from build123d import *

# Parameters (mm, degrees)
F0_W     = 1044
F0_H     = 389
F1_DEPTH = 288
F2_R     = 100
F4_DEPTH = 389.001
F5_R     = 15
F6_DEPTH = 50


with BuildPart() as f1:
    # F0 (on Front) → F1 (new body)
    with BuildSketch(Plane.XZ):
        with Locations((12.094161, 0)):
            Rectangle(F0_W, F0_H)
    extrude(amount=-F1_DEPTH)

    # F2
    f2_edges = [f1.edges().sort_by_distance(p)[0] for p in [
        (-509.905839, 144, 194.5),
        (-509.905839, 288, 0),
        (-509.905839, 144, -194.5),
        (-509.905839, 0, 0),
    ]]
    fillet(f2_edges, radius=F2_R)

    # F3 (on face) → F4 (cut, through all)
    with BuildSketch(Plane.XY.offset(194.5)):
        Polygon((534.094161, 288), (332.893832, 288), (534.094161, 194.178746), align=None)
    extrude(amount=-F4_DEPTH, mode=Mode.SUBTRACT)

    # F5 (on face) → F6 (join)
    with BuildSketch(Plane.XZ):
        with Locations((162.094161, -163.5)):
            Circle(F5_R)
        with Locations((-308.905839, -163.5)):
            Circle(F5_R)
        with Locations((162.094161, 163.5)):
            Circle(F5_R)
        with Locations((-308.905839, 163.5)):
            Circle(F5_R)
    extrude(amount=F6_DEPTH)


with BuildPart() as f1_1:
    # F7: moved
    add(f1.part.moved(Location((0, 50, 0))))


solid = f1_1.part
Source: CAD feature listing. Evaluate the final solid. Frame: model axes, mm. A direction names the side the tool comes from. Coordinates: 2 decimals unless noted, no trailing zeros. Order: outer loops, then holes, each group sorted by start corner. A loop starts at its lowest first (then second) coordinate and runs counter-clockwise, first axis right, second up. Notation, with made-up numbers: M 27.25,64 L 85.25,64 A31 ccw 85.25,89 Z; hole C 76.5,40 d11. An arc over 180 degrees is marked long. Write each question's results on one line, items separated by ' | '. Start each with the question number.
Item 1: Cut plane D-D (z = 6.5). Return loops of the section in (x, y), and give its area (3 significant figures).
Item 2: Set-up query: faces 1 (the face through (55, 192, -194.5)), 2 (the face through (-320.809, 25.35, 154.373)). Return all of +Z, -Z, +X, -X, +Y, -Y with unobstructed straight access to the full face (end or side cutting, diameter ignored); none if empty.
Item 3: Cut plane A-A (z = -163.5). Return loops of the section in (x, y).
Item 4: Cut plane C-C (x = -195.5). Return loops of the section in (y, z).
Item 5: First-contact query: pin 1 Ø5 at (x, z) = (-196, -1) entering from -Y; pin 2 Ø8 at (y, z) = (248.5, 137.5) entering from -X. Flat tips, straight axial feed; report the tip coordinate or a pass-through.
Item 6: Line query: probe 1 along Y at (x, z) = (-196, 172); probe 2 along X at (y, z) = (31, 167); probe 3 along X at (y, z) = (299.5, -112). Output: solid intervals per line, ascending.
Item 7: Draft query along X for faces 3 (the face through (-468.16, 319.28, 2.72)), 4 (the face through (162, 0, -163)), 5 (the face through (175.95, 25.35, -169.25)). Return one class per face: pulls with the +X half, pulls with the -X half, needs draft (parallel to the pull), parting line crosses it, or undercut.
Item 8: Cut plane B-B (y = 36). Return loops of the section in (x, z), and give its area (3 significant figures).
Checked values:
1) outline: M -509.91,150 A100 ccw -409.91,50 L 534.09,50 L 534.09,244.18 L 332.89,338 L -409.91,338 A100 ccw -509.91,238 Z | area: 287,000 mm2
2) face 1: -Z, +X, -X, +Y, -Y | face 2: -Y
3) outline: M -482.29,81 A100 ccw -409.91,50 L -323.91,50 L -323.91,0 L -293.91,0 L -293.91,50 L 147.09,50 L 147.09,0 L 177.09,0 L 177.09,50 L 534.09,50 L 534.09,244.18 L 332.89,338 L -409.91,338 A100 ccw -482.29,307 Z
4) outline: M 50,-194.5 L 338,-194.5 L 338,194.5 L 50,194.5 Z
5) pin 1: stops at y = 50 | pin 2: stops at x = -501.99
6) probe 1: y = 50 to 338 | probe 2: x = -323.49 to -294.32, 147.51 to 176.68 | probe 3: x = -488.76 to 415.46
7) face 3: pulls with the -X half | face 4: needs draft | face 5: undercut
8) outline: C -308.91,-163.5 d30; C -308.91,163.5 d30; C 162.09,-163.5 d30; C 162.09,163.5 d30 | area: 2,830 mm2
